For this review, take the finished solid that the model builds, in its own axes (mm). Give positions to 0.01 mm unless a question says otherwise; leave off trailing zeros. Order: outer loops, then holes, each group sorted by start corner. A loop starts at its lowest first (then second) coordinate and runs counter-clockwise, first axis right, second up. Notation, with made-up numbers: (39, 11.5) -> (66, 11.5) arc R24 cw to (66, 36.5) -> close; hole circle Ø3 at (45.25, -14.5). An arc over 180 degrees is marked (long way). Return JSON: item names as keys, results as strings. Group by question number.
1) Insertion check: P1, Ø1.6, axis at x = -1.5, z = 3.5, coming from the +Y side; P2, Ø3.5, axis at x = 0, y = -65.758, coming from the -Z side; P3, Ø3, axis at y = 11.5, z = 2.5, coming from the +X side; P4, Ø8, axis at x = -65.758, y = 0, coming from the +Z side. Each pin has a flat end and moves straight along its axis. Give the tip position at first contact, or say it passes through.
2) To check wall thickness, follow line 1 along Y through (x, z) = (41, 0.6); line 2 along Y through (x, z) = (-39, 2.5); line 3 along X through (y, z) = (-19, 4). State the ranges of each line that lie inside material, in increasing order.
3) Add section A-A (y = 0). Give the boundary of the cut face in (x, z), then the cut area to 3 significant figures.
4) Add section C-C (z = 1.85). State how many separate pieces and enclosed holes the cut face has, then the cut area to 3 significant figures.
from build123d import *

# Parameters (mm, degrees)
F0_R            = 75
F1_DEPTH        = 5.4
F3_D            = 6
F3_DEPTH        = 6
F3_CSINK_D      = 8.96
F3_CSINK_ANGLE  = 90
F3_TIP          = 1.8025818571
F3_COPIES_COUNT = 8
F4_SIZE         = 2


# Not quite as in the source:
# - a pattern or mirror of a feature is missing from the dataset's text; its kind, count and spacing are read off the source's solid


with BuildPart() as f1:
    # F0 (on Top) → F1 (new body)
    with BuildSketch(Plane.XY):
        Circle(F0_R)
        with BuildLine():
            ThreePointArc((-70.5093388309, 8.3326654013), (-65.5954479473, 27.1705241697), (-55.749715835, 43.9655474137))
            Line((-55.749715835, 43.9655474137), (-44.5127719526, 38.7256744271))
            Line((-44.5127719526, 38.7256744271), (-38.7256744271, 44.5127719526))
            Line((-38.7256744271, 44.5127719526), (-43.9655474137, 55.749715835))
            ThreePointArc((-43.9655474137, 55.749715835), (-27.1705241697, 65.5954479473), (-8.3326654013, 70.5093388309))
            Line((-8.3326654013, 70.5093388309), (-4.0920959037, 58.8584698905))
            Line((-4.0920959037, 58.8584698905), (4.0920959037, 58.8584698905))
            Line((4.0920959037, 58.8584698905), (8.3326654013, 70.5093388309))
            ThreePointArc((8.3326654013, 70.5093388309), (27.1705241697, 65.5954479473), (43.9655474137, 55.749715835))
            Line((43.9655474137, 55.749715835), (38.7256744271, 44.5127719526))
            Line((38.7256744271, 44.5127719526), (44.5127719526, 38.7256744271))
            Line((44.5127719526, 38.7256744271), (55.749715835, 43.9655474137))
            ThreePointArc((55.749715835, 43.9655474137), (65.5954479473, 27.1705241697), (70.5093388309, 8.3326654013))
            Line((70.5093388309, 8.3326654013), (58.8584698905, 4.0920959037))
            Line((58.8584698905, 4.0920959037), (58.8584698905, -4.0920959037))
            Line((58.8584698905, -4.0920959037), (70.5093388309, -8.3326654013))
            ThreePointArc((70.5093388309, -8.3326654013), (65.5954479473, -27.1705241697), (55.749715835, -43.9655474137))
            Line((55.749715835, -43.9655474137), (44.5127719526, -38.7256744271))
            Line((44.5127719526, -38.7256744271), (38.7256744271, -44.5127719526))
            Line((38.7256744271, -44.5127719526), (43.9655474137, -55.749715835))
            ThreePointArc((43.9655474137, -55.749715835), (27.1705241697, -65.5954479473), (8.3326654013, -70.5093388309))
            Line((8.3326654013, -70.5093388309), (4.0920959037, -58.8584698905))
            Line((4.0920959037, -58.8584698905), (-4.0920959037, -58.8584698905))
            Line((-4.0920959037, -58.8584698905), (-8.3326654013, -70.5093388309))
            ThreePointArc((-8.3326654013, -70.5093388309), (-27.1705241697, -65.5954479473), (-43.9655474137, -55.749715835))
            Line((-43.9655474137, -55.749715835), (-38.7256744271, -44.5127719526))
            Line((-38.7256744271, -44.5127719526), (-44.5127719526, -38.7256744271))
            Line((-44.5127719526, -38.7256744271), (-55.749715835, -43.9655474137))
            ThreePointArc((-55.749715835, -43.9655474137), (-65.5954479473, -27.1705241697), (-70.5093388309, -8.3326654013))
            Line((-70.5093388309, -8.3326654013), (-58.8584698905, -4.0920959037))
            Line((-58.8584698905, -4.0920959037), (-58.8584698905, 4.0920959037))
            Line((-58.8584698905, 4.0920959037), (-70.5093388309, 8.3326654013))
        make_face(mode=Mode.SUBTRACT)
    extrude(amount=F1_DEPTH)

    # F3
    with Locations(Plane.XY.offset(5.4)):
        with Locations((-65.758, 0)):
            f3 = CounterSinkHole(F3_D / 2, F3_CSINK_D / 2, depth=F3_DEPTH, counter_sink_angle=F3_CSINK_ANGLE)
            with Locations((0, 0, -(F3_DEPTH + F3_TIP / 2))):  # 118° drill point
                Cone(0, F3_D / 2, F3_TIP, mode=Mode.SUBTRACT)

    # F3_copies: F3 ×8 about axis
    f3_copies_axis = Axis((0, 0, 0), (0, 0, 1))
    for i in range(1, F3_COPIES_COUNT):
        add(f3.rotate(f3_copies_axis, i * 360 / F3_COPIES_COUNT), mode=Mode.SUBTRACT)

    # F4
    f4_edges = [f1.edges().sort_by_distance(p)[0] for p in [
        (-75, 0, 5.4),
    ]]
    chamfer(f4_edges, length=F4_SIZE)


solid = f1.part
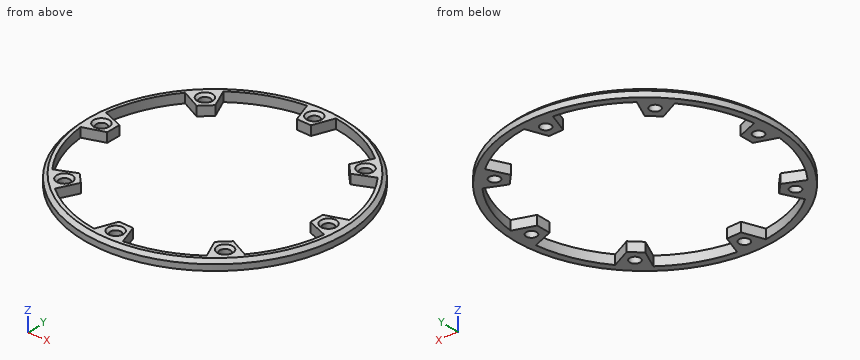
Evaluation:
{
 "1": {"P1": "y = 75", "P2": "through", "P3": "x = 74.33", "P4": "z = 4.92"},
 "2": {"line 1": "-62.8 to -57.97, -49.39 to -42.24, 42.24 to 49.39, 57.97 to 62.8", "line 2": "-64.06 to -59.33, -45.1 to -44.24, 44.24 to 45.1, 59.33 to 64.06", "line 3": "-71.93 to -68.41, 68.41 to 71.93"},
 "3": {"outline": "(-75, 0) -> (-68.76, 0) -> (-68.76, 3.92) -> (-70.24, 5.4) -> (-73, 5.4) -> (-75, 3.4) -> close; (-62.76, 0) -> (-58.86, 0) -> (-58.86, 5.4) -> (-61.28, 5.4) -> (-62.76, 3.92) -> close; (58.86, 0) -> (62.76, 0) -> (62.76, 3.92) -> (61.28, 5.4) -> (58.86, 5.4) -> close; (68.76, 0) -> (75, 0) -> (75, 3.4) -> (73, 5.4) -> (70.24, 5.4) -> (68.76, 3.92) -> close", "area": "101 mm^2"},
 "4": {"separate pieces": "1", "enclosed holes": "9", "area": "2,810 mm^2"}
}
